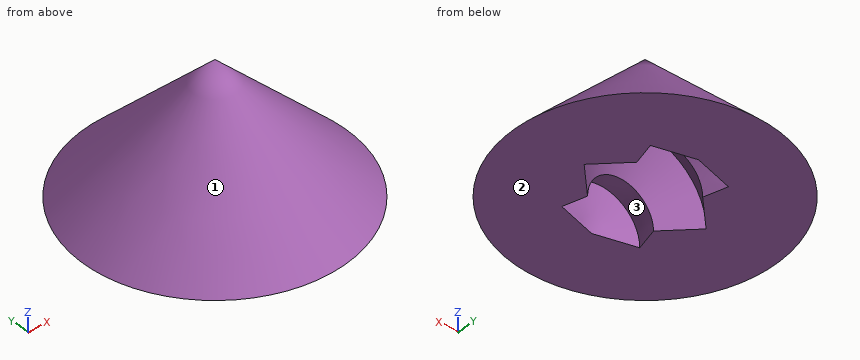
from build123d import *


with BuildPart() as f1:
    # F0 (on Front) → F1 (revolve)
    with BuildSketch(Plane.XZ):
        Polygon((53.881537, 0), (0, 53.881537), (0, 0), align=None)
    revolve(axis=Axis((0, 0, 26.940768), (0, 0, -1)))


with BuildPart() as f3:
    # F2 (on Top) → F3 (revolve)
    with BuildSketch(Plane.XY):
        Polygon((0, 25.4), (0, 0), (0, -25.4), (16.237638, -21.049138), (13.725667, -11.674333), (25.4, 0), (13.725667, 11.674333), (16.237638, 21.049138), align=None)
    revolve(axis=Axis((0, -12.7, 0), (0, -1, 0)))


with BuildPart() as f1_1:
    add(f1.part)

    # F4: cut F3
    add(f3.part, mode=Mode.SUBTRACT)


solid = f1_1.part
Can you work these out from the model? Positions are in its coordinate system, mm. Face numbers are marked on the shaded views. Give positions to 0.01 mm unless a question says otherwise; leave off trailing zeros. Write each loop counter-clockwise with the first axis right and the second up, starting at its lowest first coordinate (ties: lowest second). Pieces come first, ordered by that corner, then holes. Notation, with made-up numbers: M 48,-24 L 64,-24 A14 cw 64,-20 Z; hole C -27.5,80.25 d5. An arc over 180 degrees is marked long. Answer in a Markdown table with one row per item. Add a question column.
Item 1: For pin 1 Ø6 at (y, z) = (15.5, 13.5) entering from -X; pin 2 Ø4 at (x, z) = (-12.5, 24.5) entering from +Y; pin 3 Ø5 at (y, z) = (-13.5, 18.5) entering from -X, each with a flat end and sliding along its axis, tell me the tip position at first contact or that it passes through.
Item 2: Imagine slicing it at B-B, the plane z = 35. Write out the boundary of the cut face in (x, y).
Item 3: Please list where these lines run through material, in increasing order: L1, parallel to Y at x = 9, z = 20; L2, parallel to X at y = 3, z = 14; L3, parallel to X at y = -20, z = 14.
Item 4: We'd pull the mould along Y, two halves only. Please class the marked faces 1, 2 and 3: released by +Y, released by -Y, zero draft, split by the parting line, or undercut.
Item 5: Imagine slicing it at A-A, the plane z = 27.5. Write out the boundary of the cut face in (x, y).
Evaluation:
| question | item | result |
|---|---|---|
| 1 | pin 1 | stops at x = -40.7 |
| 1 | pin 2 | stops at y = 28.94 |
| 1 | pin 3 | stops at x = -35.55 |
| 2 | outline | C 0,0 d37.76 |
| 3 | L1 | y = -32.66 to -3.47, 3.47 to 32.66 |
| 3 | L2 | x = -39.77 to -17.49, 17.49 to 39.77 |
| 3 | L3 | x = -34.5 to -7.66, 7.66 to 34.5 |
| 4 | face 1 | split by the parting line |
| 4 | face 2 | zero draft |
| 4 | face 3 | undercut |
| 5 | outline | C 0,0 d52.76 |
